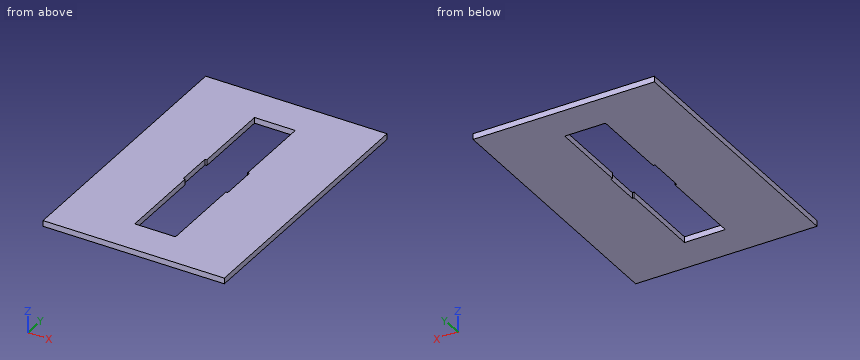
```python
from build123d import *

# Parameters (mm, degrees)
F0_W     = 200
F0_H     = 300
F1_DEPTH = 6.35
F2_W     = 2
F2_H     = 40
F3_DEPTH = 25.4


# Not quite as in the source:
# - a length typed as a fraction of an inch, garbled in the dataset ("3 / 203.2 mm" for 3/8 in), is restored


with BuildPart() as f1:
    # F0 (on Top) → F1 (new body)
    with BuildSketch(Plane.XY):
        Rectangle(F0_W, F0_H)
    extrude(amount=F1_DEPTH)

    # F2 (on face) → F3 (cut)
    with BuildSketch(Plane.XY.offset(6.35)):
        Polygon((22.5, 22.48), (22.5, 110.5), (-22.5, 110.5), (-22.5, 22.48), (-22.5, -17.52), (-22.5, -110.5), (22.5, -110.5), (22.5, -17.52), align=None)
        with Locations((23.5, 2.48)):
            Rectangle(F2_W, F2_H)
        with Locations((-23.5, 2.48)):
            Rectangle(F2_W, F2_H)
    extrude(amount=-F3_DEPTH, mode=Mode.SUBTRACT)


solid = f1.part
```
The model under review builds one solid part; all positions refer to its coordinate system, in mm. Coordinates: 2 decimals unless noted, no trailing zeros. Write each loop counter-clockwise with the first axis right and the second up, starting at its lowest first coordinate (ties: lowest second). Pieces come first, ordered by that corner, then holes. Notation, with made-up numbers: (88.25, 14) - (103.25, 14) arc R26 ccw to (103.25, 46) - close; hole circle Ø10 at (78, 46). An arc over 180 degrees is marked (long way). Answer in a Markdown table with one row per item. Add a question column.
Q1. Consider section B-B on x = -16.5. Give the boundary of the cut face in (y, z).
Q2. Consider section C-C on z = 1.75. Give the boundary of the cut face in (x, y), then the cut area to 3 significant figures.
Q3. To check wall thickness, follow line 1 along X through (y, z) = (10, 5); line 2 along X through (y, z) = (76, 5.5); line 3 along Y through (x, z) = (-24, 6.25). State the ranges of each line that lie inside material, in increasing order. Write a range as from..to.
Q4. Consider section A-A on y = -1. Give the boundary of the cut face in (x, z), then the cut area to 3 significant figures.
Answers below:
| question | item | result |
|---|---|---|
| 1 | outline | (-150, 0) - (-110.5, 0) - (-110.5, 6.35) - (-150, 6.35) - close; (110.5, 0) - (150, 0) - (150, 6.35) - (110.5, 6.35) - close |
| 2 | outline | (-100, -150) - (100, -150) - (100, 150) - (-100, 150) - close; hole (-24.5, -17.52) - (-22.5, -17.52) - (-22.5, -110.5) - (22.5, -110.5) - (22.5, -17.52) - (24.5, -17.52) - (24.5, 22.48) - (22.5, 22.48) - (22.5, 110.5) - (-22.5, 110.5) - (-22.5, 22.48) - (-24.5, 22.48) - close |
| 2 | area | 49,900 mm² |
| 3 | line 1 | -100..-24.5, 24.5..100 |
| 3 | line 2 | -100..-22.5, 22.5..100 |
| 3 | line 3 | -150..-17.52, 22.48..150 |
| 4 | outline | (-100, 0) - (-24.5, 0) - (-24.5, 6.35) - (-100, 6.35) - close; (24.5, 0) - (100, 0) - (100, 6.35) - (24.5, 6.35) - close |
| 4 | area | 959 mm² |
